Answer from the drawing. Dimensions are ordinates in mm from the lowest x, y and z of the part. Give positions to 0.01 mm unless a question says otherwise; leave off trailing zeros.
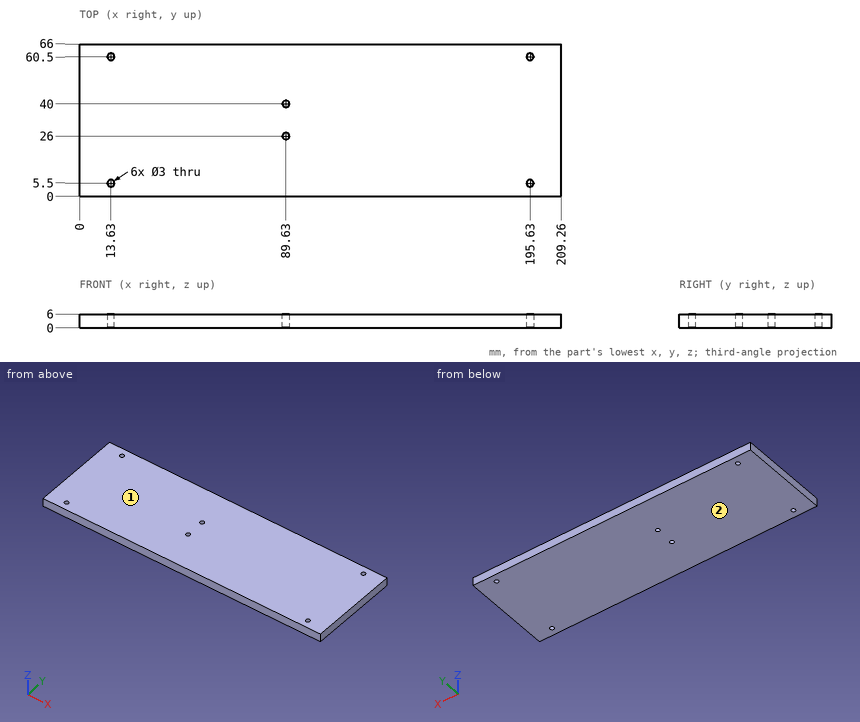
1) For a pull along Z with two mould halves and no side action, classify the marked faces 1 and 2 as released by +Z, released by -Z, zero draft, split by the parting line, or undercut.
Final values:
face 1: released by +Z
face 2: released by -Z
2) Consider L1, parallel to Y at x = 89.63, z = 3.85; L2, parallel to Y at x = 195.63, z = 3.9. Determine where each line is inside the solid, lowest interval first.
Final values:
L1: y = 0 to 24.5, 27.5 to 38.5, 41.5 to 66
L2: y = 0 to 4, 7 to 59, 62 to 66
3) Given pin 1 (2.5 mm diameter, centred on x = 89.63, y = 26, fed in from +Z), flat-ended and moving along its own axis, determine where the tip first touches the part or whether it passes through.
Final values:
pin 1: passes through
